Geometry: final body of the model. Coordinates: model frame, mm. Face numbers are marked on the shaded views. A direction names the side the tool comes from. Round coordinates to 2 decimals unless told otherwise and drop trailing zeros. Order: outer loops, then holes, each group sorted by start corner. A loop starts at its lowest first (then second) coordinate and runs counter-clockwise, first axis right, second up. Notation, with made-up numbers: (22.5, 86.5) - (72.5, 86.5) arc R28 ccw to (72.5, 121.5) - close; hole circle Ø1 at (4.5, 22). An arc over 180 degrees is marked (long way). Put each result on its own line as item: value. Start each with the question number.
(1) Section C-C (y = 22). Output: boundary loops of the cut face in (x, z), and give its area (3 significant figures).
(2) Section D-D (z = 1). Output: boundary loops of the cut face in (x, y) (3 decimals).
(3) Access query for the marked faces 1, 2 and 3. Directions: +Z, -Z, +X, -X, +Y, -Y. A direction counts if a zero-diameter tool reaches every point of the face in a straight line with its end or side. Return the directions, or none.
(4) Section B-B (x = 18.5). Output: boundary loops of the cut face in (y, z) (3 decimals), and give its area (3 significant figures).
(5) Pull-direction query (Y, two-part tool) for the marked faces 4, 5, 6 and 7; classes: released by +Y, released by -Y, zero draft, split by the parting line, or undercut.
(6) Section A-A (z = 7.25). Output: boundary loops of the cut face in (x, y) (3 decimals).
(7) Material intervals for L1, parallel to Y at x = 10, z = 7.6 (3 decimals); L2, parallel to Y at x = 10, z = 3 (3 decimals); L3, parallel to Z at x = 14, y = -21, sorted ascending. Write a range as [from, to].
(8) Pin query (flat end, axial travel): P1, Ø5, axis at x = 5, y = -12.5, coming from the +Z side; P2, Ø11, axis at x = 8.5, y = -22.5, coming from the +Z side. Return the tip coordinate at first contact, or that it passes through.
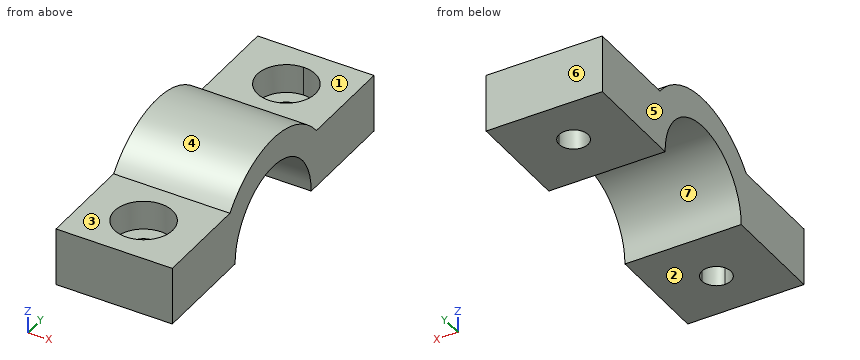
from build123d import *

# Parameters (mm, degrees)
F1_DEPTH = 20
F4_DEPTH = 5
F5_DEPTH = 25
F8_DEPTH = 5
F9_DEPTH = 25


with BuildPart() as f1:
    # F0 (on Right) → F1 (new body)
    with BuildSketch(Plane.YZ):
        with BuildLine():
            ThreePointArc((-11, 0), (0, 11), (11, 0))
            Line((11, 0), (29.125, 0))
            Line((29.125, 0), (29.125, 10))
            Line((29.125, 10), (12.4899959968, 10))
            ThreePointArc((12.4899959968, 10), (0, 16), (-12.4899959968, 10))
            Line((-12.4899959968, 10), (-29.125, 10))
            Line((-29.125, 10), (-29.125, 0))
            Line((-29.125, 0), (-11, 0))
        make_face()
    extrude(amount=F1_DEPTH)

    # F3 (on offset) → F4 (cut)
    with BuildSketch(Plane.XY.offset(10)):
        with BuildLine():
            ThreePointArc((15, -20.6245866863), (6.4644660941, -17.0890527804), (10, -25.6245866863))
            ThreePointArc((10, -25.6245866863), (13.5355339059, -24.1601205923), (15, -20.6245866863))
        make_face()
        with BuildLine():
            ThreePointArc((12.5, -20.6245866863), (11.767766953, -22.3923536393), (10, -23.1245866863))
            ThreePointArc((10, -23.1245866863), (8.232233047, -18.8568197334), (12.5, -20.6245866863))
        make_face(mode=Mode.SUBTRACT)
    extrude(amount=-F4_DEPTH, mode=Mode.SUBTRACT)

    # F3 (on offset) → F5 (cut)
    with BuildSketch(Plane.XY.offset(10)):
        with BuildLine():
            ThreePointArc((12.5, -20.6245866863), (8.232233047, -18.8568197334), (10, -23.1245866863))
            ThreePointArc((10, -23.1245866863), (11.767766953, -22.3923536393), (12.5, -20.6245866863))
        make_face()
    extrude(amount=-F5_DEPTH, mode=Mode.SUBTRACT)

    # F7 (on offset) → F8 (cut)
    with BuildSketch(Plane.XY.offset(10)):
        with BuildLine():
            ThreePointArc((15, 20.6246930474), (13.5355339059, 24.1602269533), (10, 25.6246930474))
            ThreePointArc((10, 25.6246930474), (6.4644660941, 17.0891591415), (15, 20.6246930474))
        make_face()
        with BuildLine():
            ThreePointArc((12.5, 20.6246930474), (8.232233047, 18.8569260944), (10, 23.1246930474))
            ThreePointArc((10, 23.1246930474), (11.767766953, 22.3924600004), (12.5, 20.6246930474))
        make_face(mode=Mode.SUBTRACT)
    extrude(amount=-F8_DEPTH, mode=Mode.SUBTRACT)

    # F9 (cut): a face of the model
    f9_faces = [f1.faces().sort_by_distance(p)[0] for p in [
        (10, 20.6246930474, 10),
    ]]
    extrude(f9_faces, amount=-F9_DEPTH, mode=Mode.SUBTRACT)


solid = f1.part
Checks:
1. outline: (0, 0) - (7.91, 0) - (7.91, 5) - (5.19, 5) - (5.19, 10) - (0, 10) - close; (12.09, 0) - (20, 0) - (20, 10) - (14.81, 10) - (14.81, 5) - (12.09, 5) - close
1. area: 131 mm²
2. outline: (0, -29.125) - (20, -29.125) - (20, -10.954) - (0, -10.954) - close; (0, 10.954) - (20, 10.954) - (20, 29.125) - (0, 29.125) - close; hole circle Ø5 at (10, -20.625); hole circle Ø5 at (10, 20.625)
3. face 1: +Z, +X, -X, +Y
3. face 2: -Z, +X, -X, +Y, -Y
3. face 3: +Z, +X, -X, -Y
4. outline: (-29.125, 0) - (-11, 0) arc R11 cw to (11, 0) - (29.125, 0) - (29.125, 10) - (12.49, 10) arc R16 ccw to (-12.49, 10) - (-29.125, 10) - close
4. area: 497 mm²
5. face 4: split by the parting line
5. face 5: zero draft
5. face 6: released by +Y
5. face 7: undercut
6. outline: (0, -29.125) - (20, -29.125) - (20, -8.273) - (0, -8.273) - close; (0, 8.273) - (20, 8.273) - (20, 29.125) - (0, 29.125) - close; hole circle Ø10 at (10, -20.625); hole circle Ø10 at (10, 20.625)
7. L1: y = [-29.125, -25.625], [-15.625, -7.952], [7.952, 15.625], [25.625, 29.125]
7. L2: y = [-29.125, -23.125], [-18.125, -10.583], [10.583, 18.125], [23.125, 29.125]
7. L3: z = [0, 5]
8. P1: stops at z = 12.49
8. P2: stops at z = 10
